Model file for the job. Use its own axes, mm. Face numbers are marked on the shaded views. A direction names the side the tool comes from. Give positions to 0.01 mm unless a question says otherwise; leave off trailing zeros. Loops run counter-clockwise (first coordinate to the right, second up) from the corner with the lowest first, then second, coordinate; pieces in that order, holes last. Notation, with made-up numbers: (47, -32) - (90, -32) arc R33 ccw to (90, 4) - close; hole circle Ø9 at (28, -25). An arc over 180 degrees is marked (long way). Answer as CSV lines item,"result". Start each with the question number.
Item 1: Pin check, flat tips, straight feed: pin 1 (2 mm diameter, centred on y = 1, z = 23, fed in from -X); pin 2 (1.5 mm diameter, centred on x = -2, z = 0.5, fed in from +Y); pin 3 (1.1 mm diameter, centred on y = 2, z = 1, fed in from -X). Stop position of each tip, or through.
Item 2: Drill centre lines: L1, parallel to Y at x = 0, z = 2.4; L2, parallel to Z at x = 1.8, y = 0.6; L3, parallel to Y at x = -0.1, z = 13.75. Where is each one in solid material? Low to high. Write a range as from..to.
Item 3: Saw through at A-A on z = 20. Give the cut face in (x, y).
Item 4: Tool access for the marked faces 1 and 2: list every direction of +Z, -Z, +X, -X, +Y, -Y with a clear straight run to the whole face (end or side of a thin tool).
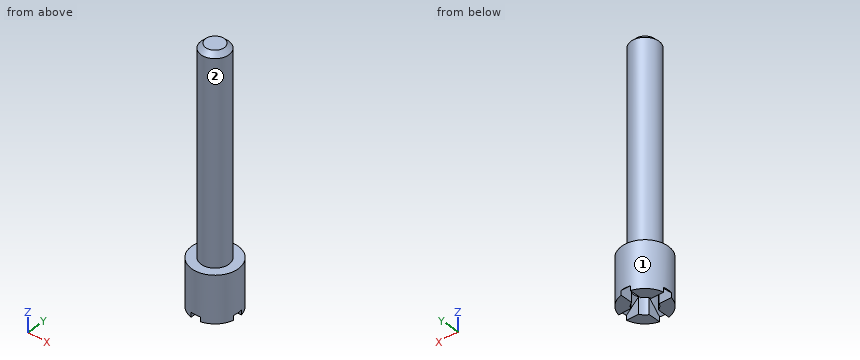
Autodesk Inventor part; units mm, degrees
ref_plane "YZ Plane" through (0, 0, 0) normal (1, 0, 0) x (0, 1, 0)
ref_plane "XZ Plane" through (0, 0, 0) normal (0, 1, 0) x (-1, 0, 0)
ref_plane "XY Plane" through (0, 0, 0) normal (0, 0, 1) x (1, 0, 0)
sketch "Esboço1" plane through (0, 0, 0) normal (0, 0, 1) x (1, 0, 0)
  circle A0 centre (0, 0) radius 2.5
  dimension "d0" = 5
extrude "Extrusão1" add sketch "Esboço1" along normal blind 5
sketch "Esboço2" plane through (0, 0, 5) normal (0, 0, 1) x (1, 0, 0)
  circle A0 centre (0, 0) radius 1.5
  dimension "d3" = 3
extrude "Extrusão2" add sketch "Esboço2" along normal blind 22
thread "Rosca1"
sketch "Esboço3" plane through (0, 0, 0) normal (0, 0, -1) x (-1, 0, 0)
  point P0 (0, 0)
  point P1 (0, 0)
  dimension "d15" = 0
  dimension "d16" = 0
hole "Furo1" at (0, 0, 0) direction (0, 0, 1) diameter 2.459 depth 4 tip angle 118
sketch "Esboço4" plane through (0, 0, 0) normal (0, 0, -1) x (-1, 0, 0)
  line L0 (-0.5, -3) -> (0.5, -3)
  line L1 (0.5, -3) -> (0.5, 3)
  line L2 (0.5, 3) -> (-0.5, 3)
  line L3 (-0.5, 3) -> (-0.5, -3)
  line L4 (-0.5, -3) -> (0.5, 3) construction
  line L5 (0.5, -3) -> (-0.5, 3) construction
  line L6 (-3, -0.5) -> (3, -0.5)
  line L7 (3, -0.5) -> (3, 0.5)
  line L8 (3, 0.5) -> (-3, 0.5)
  line L9 (-3, 0.5) -> (-3, -0.5)
  line L10 (-3, -0.5) -> (3, 0.5) construction
  line L11 (3, -0.5) -> (-3, 0.5) construction
  point P0 (0, 0)
  point P1 (-0.5, -0.5)
  point P2 (-0.5, 0.5)
  point P3 (0.5, 0.5)
  point P4 (0.5, -0.5)
  dimension "d17" = 1
  dimension "d18" = 6
  dimension "d19" = 6
  dimension "d20" = 1
extrude "Extrusão3" cut sketch "Esboço4" against normal blind 0.5 contours L3 L6 L1 L0 | L6 L9 L8 L3 | L1 L8 L7 L6 | L3 L2 L1 L8
chamfer "Chanfro1" distance 1.27 angle 45 3 edges at (0, -1.2295, 0.5) (1.2295, 0, 0.5) (-1.2295, 0, 0.5)
chamfer "Chanfro2" distance 0.5 angle 45 1 edges at (-1.5, 0, 27)
properties part number "PARAFUSO"
Responses:
1,pin 1,"x = -1.5"
1,pin 2,"y = 2.17"
1,pin 3,"x = -2.04"
2,L1,"-2.5..-1.23, 1.23..2.5"
2,L2,"0..5"
2,L3,"-1.5..1.5"
3,outline,"circle Ø3 at (0, 0)"
4,face 1,"+Z, -Z"
4,face 2,"+Z"
